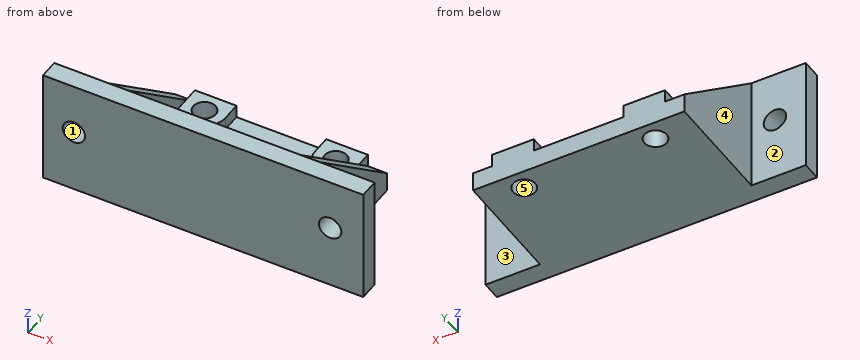
```python
from build123d import *

# Parameters (mm, degrees)
CROQUIS1_W              = 33
CROQUIS1_H              = 21
CROQUIS1_R              = 1.75
SALIENTE_EXTRUIR1_DEPTH = 3
SALIENTE_EXTRUIR2_DEPTH = 15
CORTAR_EXTRUIR1_DEPTH   = 44.058100283
CROQUIS4_W              = 8.5
CROQUIS4_H              = 18
SALIENTE_EXTRUIR3_DEPTH = 3
CROQUIS5_R              = 1.75
SALIENTE_EXTRUIR4_DEPTH = 2
CROQUIS8_R              = 1.75
CORTAR_EXTRUIR4_DEPTH   = 50.872337022


with BuildPart() as part:
    # Croquis1 → Saliente-Extruir1 (new body)
    with BuildSketch(Plane.XY):
        with Locations((16.5, -10.5)):
            Rectangle(CROQUIS1_W, CROQUIS1_H)
        with Locations((6.25, -3)):
            Circle(CROQUIS1_R, mode=Mode.SUBTRACT)
        with Locations((26.75, -3)):
            Circle(CROQUIS1_R, mode=Mode.SUBTRACT)
    extrude(amount=SALIENTE_EXTRUIR1_DEPTH)

    # Croquis2 → Saliente-Extruir2 (add)
    with BuildSketch(Plane.XY.offset(3)):
        Polygon((0, 0), (0, -21), (33, -21), (33, 0), (30, 0), (30, -18), (3, -18), (3, 0), align=None)
    extrude(amount=SALIENTE_EXTRUIR2_DEPTH)

    # Croquis3 → Cortar-Extruir1 (cut, through all)
    with BuildSketch(Plane.ZY):
        Polygon((3, 0), (18, -18), (18, 0), align=None)
    extrude(amount=-CORTAR_EXTRUIR1_DEPTH, mode=Mode.SUBTRACT)

    # Croquis4 → Saliente-Extruir3 (add)
    with BuildSketch(Plane(origin=(0, -18, 0), x_dir=(1, 0, 0), z_dir=(0, 1, 0))):
        with Locations((-4.25, -9)):
            Rectangle(CROQUIS4_W, CROQUIS4_H)
        with Locations((37.25, -9)):
            Rectangle(CROQUIS4_W, CROQUIS4_H)
    extrude(amount=-SALIENTE_EXTRUIR3_DEPTH)

    # Croquis5 → Saliente-Extruir4 (add)
    # profile 1 of 2: a face of its own
    with BuildSketch(Plane.XY.offset(3)):
        with BuildLine():
            Line((6.25, -6.25), (3, -6.25))
            Line((3, -6.25), (3, 0))
            Line((3, 0), (9.5, 0))
            Line((9.5, 0), (9.5, -3))
            ThreePointArc((9.5, -3), (8.548097039, -5.298097039), (6.25, -6.25))
        make_face()
        with Locations((6.25, -3)):
            Circle(CROQUIS5_R, mode=Mode.SUBTRACT)
    # profile 2 of 2: a face of its own
    with BuildSketch(Plane.XY.offset(3)):
        with BuildLine():
            Line((23.5, 0), (23.5, -3))
            ThreePointArc((23.5, -3), (24.451902961, -5.298097039), (26.75, -6.25))
            Line((26.75, -6.25), (30, -6.25))
            Line((30, -6.25), (30, 0))
            Line((30, 0), (23.5, 0))
        make_face()
        with Locations((26.75, -3)):
            Circle(CROQUIS5_R, mode=Mode.SUBTRACT)
    extrude(amount=SALIENTE_EXTRUIR4_DEPTH)

    # Croquis8 → Cortar-Extruir4 (cut, through all)
    with BuildSketch(Plane.XZ.offset(21)):
        with Locations(Location((-3.675, 10, 0), (0, 0, 270))):
            Circle(CROQUIS8_R)
        with Locations(Location((36.325, 10, 0), (0, 0, 270))):
            Circle(CROQUIS8_R)
    extrude(amount=-CORTAR_EXTRUIR4_DEPTH, mode=Mode.SUBTRACT)


solid = part.part
```
Work out the finished part from the listing and answer in its coordinate system (mm). Face numbers are marked on the shaded views. A direction names the side the tool comes from. Coordinates: 2 decimals unless noted, no trailing zeros. Order: outer loops, then holes, each group sorted by start corner. A loop starts at its lowest first (then second) coordinate and runs counter-clockwise, first axis right, second up. Notation, with made-up numbers: (-15.75, -10) - (-5.75, -10) arc R23 cw to (-5.75, 12) - close; hole circle Ø7 at (89.25, 21). An arc over 180 degrees is marked (long way). Answer as a JSON object with one key per item and string values.
1. Find section D-D on z = 13. Determine the outline of the cut face in (x, y), plus the area to 3 significant figures.
Output values:
{"outline": "(-8.5, -21) - (41.5, -21) - (41.5, -18) - (33, -18) - (33, -12) - (30, -12) - (30, -18) - (3, -18) - (3, -12) - (0, -12) - (0, -18) - (-8.5, -18) - close", "area": "186 mm²"}
2. Consider line 1 (X direction, y = -19.55, z = 10) (3 decimals); line 2 (X direction, y = -14.75, z = 11.5); line 3 (Y direction, x = 6.25, z = 1.35). Determine where each line is inside the solid, lowest interval first.
Output values:
{"line 1": "x = -8.5 to -5.425, -1.925 to 34.575, 38.075 to 41.5", "line 2": "x = 0 to 3, 30 to 33", "line 3": "y = -21 to -4.75, -1.25 to 0"}
3. Each of these flat-tipped pins is pushed along its axis until it touches: P1, Ø2, axis at y = -1, z = 4.5, coming from the +X side; P2, Ø1.6, axis at y = -1, z = 4, coming from the -X side; P3, Ø5, axis at x = 14, z = 14, coming from the +Y side. Where does it stop, or does it pass through?
Output values:
{"P1": "stops at x = 33", "P2": "stops at x = 0", "P3": "stops at y = -18"}
4. A tool of negligible diameter and unlimited length cuts with its end or side. For the marked faces 1 and 2, from which of +Z, -Z, +X, -X, +Y, -Y can it reach the whole face along a straight path? Write none if from no direction.
Output values:
{"face 1": "+Y, -Y", "face 2": "+Z, -Z, -X, +Y"}
5. The mould has two halves that part along X. Classify the marked faces 3, 4 and 5: +X half, -X half, draft (parallel to the pull), parting line (faces both ways), or undercut.
Output values:
{"face 3": "draft", "face 4": "-X half", "face 5": "undercut"}
6. Find section B-B on x = -2.5. Determine the outline of the cut face in (y, z), plus the area to 3 significant figures.
Output values:
{"outline": "(-21, 0) - (-18, 0) - (-18, 8.7) - (-21, 8.7) - close; (-21, 11.3) - (-18, 11.3) - (-18, 18) - (-21, 18) - close", "area": "46.2 mm²"}
7. Find section A-A on z = 10. Determine the outline of the cut face in (x, y) (3 decimals).
Output values:
{"outline": "(-8.5, -21) - (-5.425, -21) - (-5.425, -18) - (-8.5, -18) - close; (-1.925, -21) - (34.575, -21) - (34.575, -18) - (33, -18) - (33, -8.4) - (30, -8.4) - (30, -18) - (3, -18) - (3, -8.4) - (0, -8.4) - (0, -18) - (-1.925, -18) - close; (38.075, -21) - (41.5, -21) - (41.5, -18) - (38.075, -18) - close"}
8. Find section C-C on x = 18.5. Determine the outline of the cut face in (y, z), plus the area to 3 significant figures.
Output values:
{"outline": "(-21, 0) - (0, 0) - (0, 3) - (-18, 3) - (-18, 18) - (-21, 18) - close", "area": "108 mm²"}
